from build123d import *

# Parameters (mm, degrees)
SKETCH1_W           = 67.00000001
SKETCH1_H           = 37.49999993
BOSS_EXTRUDE1_DEPTH = 1.524
SKETCH2_W           = 45.085000006
SKETCH2_H           = 31.496000001
BOSS_EXTRUDE2_DEPTH = 16.9418
HOLE1_D             = 3.048
HOLE2_D             = 3.048
HOLE2_DEPTH         = 18.4658
HOLE3_D             = 3.048
HOLE3_DEPTH         = 18.4658
HOLE4_D             = 3.048
HOLE4_DEPTH         = 18.4658
FILLET1_R           = 2.54


with BuildPart() as part:
    # Sketch1 → Boss-Extrude1 (new body)
    with BuildSketch(Plane(origin=(0, 0, 0), x_dir=(-1, 0, 0), z_dir=(0, 0, -1))):
        Rectangle(SKETCH1_W, SKETCH1_H)
    extrude(amount=-BOSS_EXTRUDE1_DEPTH)

    # Sketch2 → Boss-Extrude2 (add)
    with BuildSketch(Plane.XY.offset(1.524)):
        with Locations((-2.067500005, 2.112999961)):
            Rectangle(SKETCH2_W, SKETCH2_H)
    extrude(amount=BOSS_EXTRUDE2_DEPTH)

    # Hole1 (through all)
    with Locations(Plane.XY.offset(1.524)):
        with Locations((31.015999995, -16.556000035)):
            Hole(HOLE1_D / 2)

    # Hole2
    with Locations(Plane(origin=(0, 0, 0), x_dir=(-1, 0, 0), z_dir=(0, 0, -1))):
        with Locations((31.214000005, -16.556000035)):
            Hole(HOLE2_D / 2, depth=HOLE2_DEPTH)

    # Hole3
    with Locations(Plane(origin=(0, 0, 0), x_dir=(-1, 0, 0), z_dir=(0, 0, -1))):
        with Locations((-31.015999995, 16.463999965)):
            Hole(HOLE3_D / 2, depth=HOLE3_DEPTH)

    # Hole4
    with Locations(Plane(origin=(0, 0, 0), x_dir=(-1, 0, 0), z_dir=(0, 0, -1))):
        with Locations((31.214000005, 16.463999965)):
            Hole(HOLE4_D / 2, depth=HOLE4_DEPTH)

    # Fillet1
    fillet1_edges = [part.edges().sort_by_distance(p)[0] for p in [
        (20.474999998, 2.112999962, 18.4658),
        (-2.067500005, 17.860999962, 18.4658),
        (-24.610000008, 2.112999962, 18.4658),
        (-2.067500005, -13.635000039, 18.4658),
    ]]
    fillet(fillet1_edges, radius=FILLET1_R)


solid = part.part
Could you check a few things on this model? Use its own coordinates, in mm. A direction names the side the tool comes from. Give positions to 0.01 mm unless a question says otherwise; leave off trailing zeros. Loops run counter-clockwise (first coordinate to the right, second up) from the corner with the lowest first, then second, coordinate; pieces in that order, holes last. Notation, with made-up numbers: (36, 43.25) -> (62, 43.25) arc R26 ccw to (62, 63.25) -> close; hole circle Ø5 at (30, 80). An arc over 180 degrees is marked (long way). Answer as CSV lines item,"result". Start each with the question number.
(1) I'm going to push flat-ended pins straight in: pin 1 Ø2.5 at (x, y) = (-31.214, -16.556) entering from +Z; pin 2 Ø4 at (x, y) = (31.016, -16.556) entering from +Z; pin 3 Ø6 at (x, z) = (-24.5, 8.5) entering from -Y (3 decimals); pin 4 Ø10 at (x, z) = (0, 15) entering from +Y. Where does each tip first touch, or does it pass through?
(2) I need wall thicknesses on probe 1 along X at (y, z) = (5.5, 10.5) (3 decimals); probe 2 along Z at (x, y) = (-27, -7); probe 3 along Y at (x, z) = (0.5, 6) (3 decimals). Which ranges of each line are inside material? Lowest first, please.
(3) If we section it at C-C on z = 14: Write out the boundary of the cut face in (x, y) (3 decimals), then the cut area to 3 significant figures.
(4) If we section it at B-B on y = 10: Write out the boundary of the cut face in (x, z) (3 decimals).
(5) We'd pull the mould along X, two halves only. Please class faces 1 (the flat face through (20.475, 2, 9)), 2 (the cylindrical face through (-23.89, 2.33, 17.7)), 3 (the cylindrical face through (-1.75, -12.91, 17.7)), 4 (the cylindrical face through (32.139, -15.526, 0.751)): released by +X, released by -X, zero draft, split by the parting line, or undercut.
(6) If we section it at D-D on x = -26.5: Write out the boundary of the cut face in (y, z).
(7) Which directions (+Z, -Z, +X, -X, +Y, -Y) give clear straight access to the entire face, cutting with the end or side of a thin tool? Please do faces 5 (the cylindrical face through (-29.76, 16.92, 0.77)), 6 (the flat face through (-24.61, 2, 9)), 7 (the flat face through (-2, -13.635, 9)).
(8) If we section it at A-A on x = -8: Write out the boundary of the cut face in (y, z) (3 decimals).
Computed:
1,pin 1,"passes through"
1,pin 2,"stops at z = 1.52"
1,pin 3,"stops at y = -13.635"
1,pin 4,"stops at y = 17.86"
2,probe 1,"x = -24.61 to 20.475"
2,probe 2,"z = 0 to 1.52"
2,probe 3,"y = -13.635 to 17.861"
3,outline,"(-24.61, -13.635) -> (20.475, -13.635) -> (20.475, 17.861) -> (-24.61, 17.861) -> close"
3,area,"1,420 mm2"
4,outline,"(-33.5, 0) -> (33.5, 0) -> (33.5, 1.524) -> (20.475, 1.524) -> (20.475, 15.926) arc R2.54 ccw to (17.935, 18.466) -> (-22.07, 18.466) arc R2.54 ccw to (-24.61, 15.926) -> (-24.61, 1.524) -> (-33.5, 1.524) -> close"
5,face 1,"released by +X"
5,face 2,"released by -X"
5,face 3,"zero draft"
5,face 4,"undercut"
6,outline,"(-18.75, 0) -> (18.75, 0) -> (18.75, 1.52) -> (-18.75, 1.52) -> close"
7,face 5,"+Z, -Z"
7,face 6,"+Z, -X, +Y, -Y"
7,face 7,"+Z, +X, -X, -Y"
8,outline,"(-18.75, 0) -> (18.75, 0) -> (18.75, 1.524) -> (17.861, 1.524) -> (17.861, 15.926) arc R2.54 ccw to (15.321, 18.466) -> (-11.095, 18.466) arc R2.54 ccw to (-13.635, 15.926) -> (-13.635, 1.524) -> (-18.75, 1.524) -> close"
